Model file for the job. Use its own axes, mm. Face numbers are marked on the shaded views. Round coordinates to 2 decimals unless told otherwise and drop trailing zeros. Order: outer loops, then holes, each group sorted by start corner. A loop starts at its lowest first (then second) coordinate and runs counter-clockwise, first axis right, second up. Notation, with made-up numbers: (-5, 69) - (8, 69) arc R19 ccw to (8, 73) - close; hole circle Ø6 at (75, 2). An arc over 180 degrees is marked (long way). Answer as CSV lines item,"result". Start each with the question number.
1. Band-saw the part on A-A on x = 0. List the corners of the cut face in (y, z), then the cut area to 3 significant figures.
2. Band-saw the part on B-B on z = 0. List the corners of the cut face in (x, y).
3. Pin check, flat tips, straight feed: pin 1 Ø8 at (x, y) = (-8, 5.5) entering from +Z; pin 2 Ø6 at (y, z) = (-8.5, 6) entering from +X; pin 3 Ø6 at (y, z) = (9.5, -7) entering from -X. Stop position of each tip, or through.
4. Pull direction X, two halves, no side cores. Call the marked faces 1, 2 and 3: released by +X, released by -X, zero draft, split by the parting line, or undercut.
5. Wall check: line 1 along X through (y, z) = (5.75, 0); line 2 along X through (y, z) = (-8.75, 5.25); line 3 along Z through (x, y) = (-1.25, 1). Give the ranges that are in metal, low to high. Write a range as [from, to].
6. Band-saw the part on C-C on y = -2.5. List the corners of the cut face in (x, z), then the cut area to 3 significant figures.
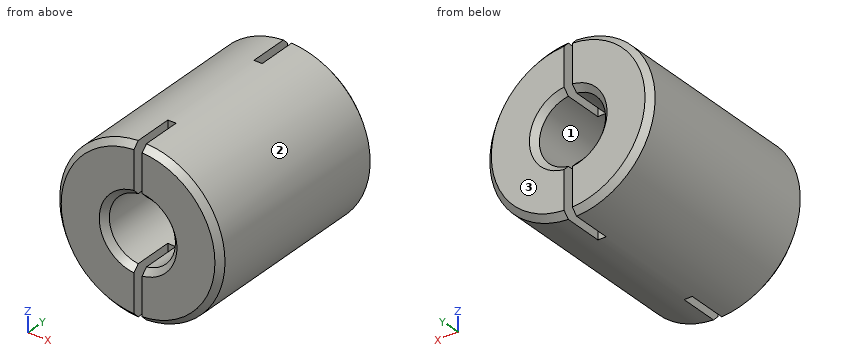
```python
from build123d import *

# Parameters (mm, degrees)
SKETCH1_R               = 10
SKETCH1_R_2             = 4
BOSS_EXTRUDE1_DEPTH     = 12.5
CHAMFER1_SIZE           = 0.7
SKETCH2_W               = 1
SKETCH2_H               = 20.36289329
CUT_EXTRUDE1_DEPTH      = 40
CUT_EXTRUDE1_DEPTH_BACK = 36


with BuildPart() as part:
    # Sketch1 → Boss-Extrude1 (new body, symmetric)
    with BuildSketch(Plane(origin=(0, 0, 0), x_dir=(1, 0, 0), z_dir=(0, 1, 0))):
        Circle(SKETCH1_R)
        Circle(SKETCH1_R_2, mode=Mode.SUBTRACT)
    extrude(amount=BOSS_EXTRUDE1_DEPTH, both=True)

    # Chamfer1
    chamfer1_edges = [part.edges().sort_by_distance(p)[0] for p in [
        (-10, -12.5, 0),
        (-10, 12.5, 0),
        (-4, -12.5, 0),
        (-4, 12.5, 0),
    ]]
    chamfer(chamfer1_edges, length=CHAMFER1_SIZE)

    # Sketch2 → Cut-Extrude1 (cut, two sides)
    with BuildSketch(Plane.XY) as cut_extrude1_sk:
        with Locations((0, 17.181446645)):
            Rectangle(SKETCH2_W, SKETCH2_H)
        with Locations((0, -17.181446645)):
            Rectangle(SKETCH2_W, SKETCH2_H)
    extrude(amount=CUT_EXTRUDE1_DEPTH, mode=Mode.SUBTRACT)
    extrude(cut_extrude1_sk.sketch, amount=-CUT_EXTRUDE1_DEPTH_BACK, mode=Mode.SUBTRACT)


solid = part.part
```
Reply:
1,outline,"(-7, -10) - (7, -10) - (7, -4) - (-7, -4) - close; (-7, 4) - (7, 4) - (7, 10) - (-7, 10) - close"
1,area,"168 mm2"
2,outline,"(-10, -11.8) - (-9.3, -12.5) - (-4.7, -12.5) - (-4, -11.8) - (-4, 11.8) - (-4.7, 12.5) - (-9.3, 12.5) - (-10, 11.8) - close; (4, -11.8) - (4.7, -12.5) - (9.3, -12.5) - (10, -11.8) - (10, 11.8) - (9.3, 12.5) - (4.7, 12.5) - (4, 11.8) - close"
3,pin 1,"stops at z = 9.17"
3,pin 2,"stops at x = 9.54"
3,pin 3,"stops at x = -9.17"
4,face 1,"undercut"
4,face 2,"split by the parting line"
4,face 3,"zero draft"
5,line 1,"x = [-10, -4], [4, 10]"
5,line 2,"x = [-8.51, -0.5], [0.5, 8.51]"
5,line 3,"z = [-9.92, -3.8], [3.8, 9.92]"
6,outline,"circle Ø20 at (0, 0); hole circle Ø8 at (0, 0)"
6,area,"264 mm2"
